Model file for the job. Use its own axes, mm. Face numbers are marked on the shaded views. A direction names the side the tool comes from. Coordinates: 2 decimals unless noted, no trailing zeros. Write each loop counter-clockwise with the first axis right and the second up, starting at its lowest first coordinate (ties: lowest second). Pieces come first, ordered by that corner, then holes. Notation, with made-up numbers: M 27,-1.75 L 80,-1.75 A22 ccw 80,36.25 Z; hole C -17,73.5 d1. An arc over 180 degrees is marked long. Put each result on its own line as item: value. Start each with the question number.
Q1. Which spindle directions (+Z, -Z, +X, -X, +Y, -Y) get a long thin tool onto all of the face, cutting with end or side? Do the marked faces 1 and 2. Say none if no direction does.
Q2. Drill centre lines: line 1 along Z through (x, y) = (10, -11); line 2 along Y through (x, z) = (5.75, 61); line 3 along Y through (x, z) = (2, 45). Where is each one in solid material? Low to high.
Q3. Cut at B-B (y = 0). Write the cut outline in (x, z), then the cut area to 3 significant figures.
Q4. Drop flat-ended pins along their axis: pin 1 (8 mm diameter, centred on x = -10, z = 39.5, fed in from +Y); pin 2 (6 mm diameter, centred on x = 2, z = 58.5, fed in from -Y); pin 3 (4 mm diameter, centred on x = -3.5, y = 31, fed in from +Z). Give the stop position or say it passes through.
Q5. Cut at C-C (y = 15.5). Write the cut outline in (x, z), then the cut area to 3 significant figures.
Q6. Cut at A-A (x = 0). Write the cut outline in (y, z), then the cut area to 3 significant figures.
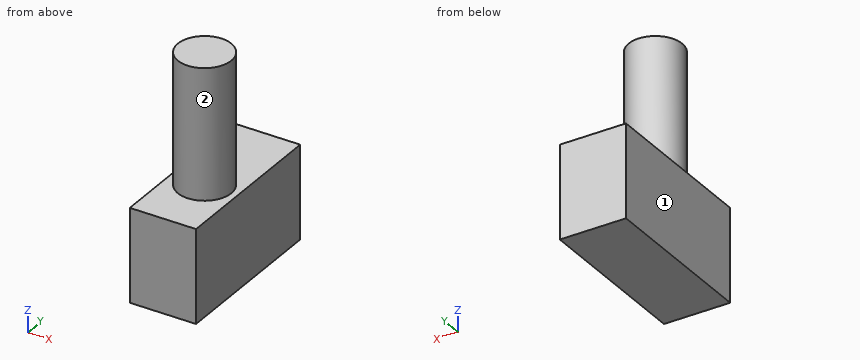
```python
from build123d import *

# Parameters (mm, degrees)
F0_W     = 25.4
F0_H     = 25.4
F1_DEPTH = 25.4
F2_DEPTH = 38.1
F3_DEPTH = 10.414
F4_R     = 10.2474826173
F5_DEPTH = 73.152


# Not quite as in the source:
# - the program builds the solid bodies; features that only make, move or delete a surface that nothing else refers to are left out


with BuildPart() as f1:
    # F0 (on Front) → F1 (new body)
    with BuildSketch(Plane.XZ):
        Rectangle(F0_W, F0_H)
    extrude(amount=F1_DEPTH)

    # F2 (add): a face of the model
    f2_faces = [f1.faces().sort_by_distance(p)[0] for p in [
        (0, 0, 0),
    ]]
    extrude(f2_faces, amount=F2_DEPTH)

    # F3 (add): a face of the model
    f3_faces = [f1.faces().sort_by_distance(p)[0] for p in [
        (0, 6.35, 12.7),
    ]]
    extrude(f3_faces, amount=F3_DEPTH)

    # F4 (on Top) → F5 (join)
    with BuildSketch(Plane.XY):
        Circle(F4_R)
    extrude(amount=F5_DEPTH)


solid = f1.part
```
Computed values:
1. face 1: +Z, -Z, -X, +Y, -Y
1. face 2: +Z
2. line 1: -12.7 to 23.11
2. line 2: -8.48 to 8.48
2. line 3: -10.05 to 10.05
3. outline: M -12.7,-12.7 L 12.7,-12.7 L 12.7,23.11 L 10.25,23.11 L 10.25,73.15 L -10.25,73.15 L -10.25,23.11 L -12.7,23.11 Z
3. area: 1,940 mm2
4. pin 1: y = 8.31
4. pin 2: y = -10.25
4. pin 3: z = 23.11
5. outline: M -12.7,-12.7 L 12.7,-12.7 L 12.7,23.11 L -12.7,23.11 Z
5. area: 910 mm2
6. outline: M -25.4,-12.7 L 38.1,-12.7 L 38.1,23.11 L 10.25,23.11 L 10.25,73.15 L -10.25,73.15 L -10.25,23.11 L -25.4,23.11 Z
6. area: 3,300 mm2
